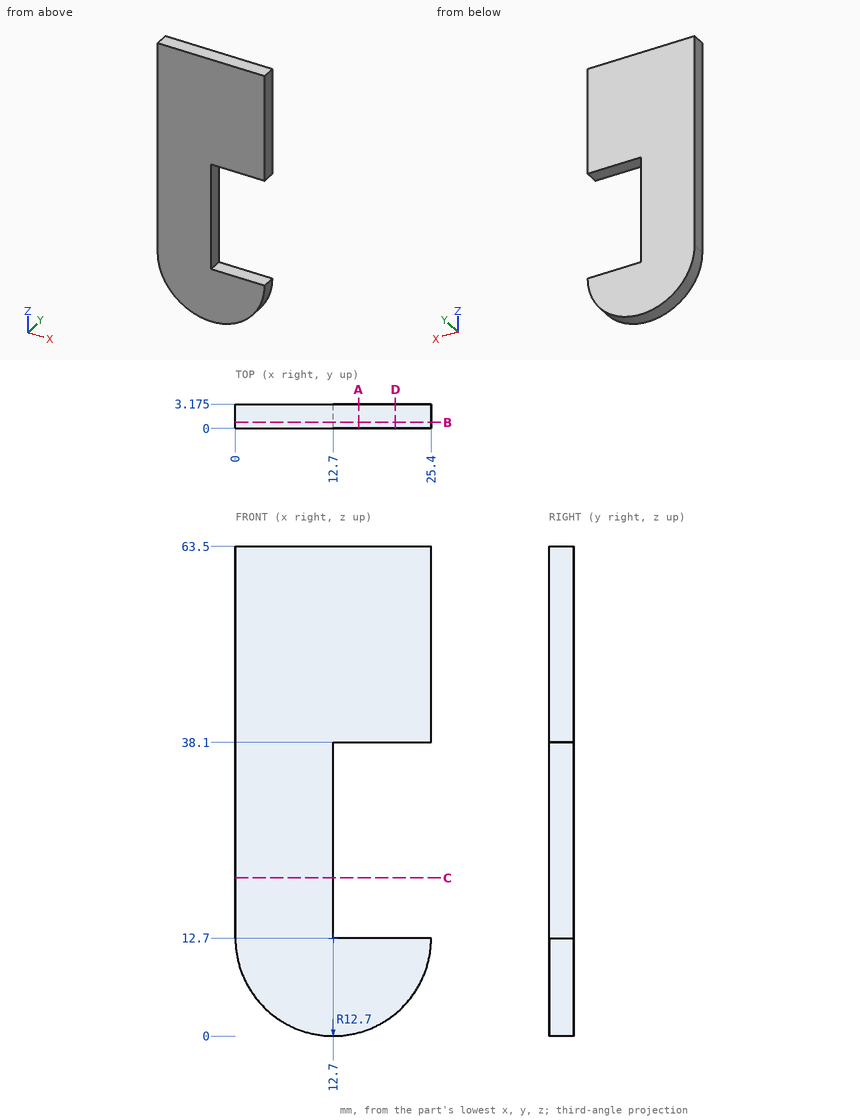
Source: three-view drawing plus pictorial views. Frame: mm from the lowest corner of the part. Round coordinates to 2 decimals unless told otherwise and drop trailing zeros. Order: outer loops, then holes, each group sorted by start corner. A loop starts at its lowest first (then second) coordinate and runs counter-clockwise, first axis right, second up. Notation, with made-up numbers: (83.25, 52) -> (125.25, 52) arc R12 cw to (125.25, 56) -> close; hole circle Ø8 at (64.5, 83). An arc over 180 degrees is marked (long way). Use one line per item in the form item = value.
(1) Ray query, probe 1 along Z at (x, y) = (19, 2.05); probe 2 along Z at (x, y) = (14, 1.4); probe 3 along X at (y, z) = (0.9, 15). Return the intervals inside material, ascending. Write a range as [from, to].
Results list:
probe_1 = [1.67, 12.7], [38.1, 63.5]
probe_2 = [0.07, 12.7], [38.1, 63.5]
probe_3 = [0, 12.7]
(2) Section A-A on x = 16. Return loops of the section in (y, z) (3 decimals), and give its area (3 significant figures).
Results list:
outline = (0, 0.436) -> (3.175, 0.436) -> (3.175, 12.7) -> (0, 12.7) -> close; (0, 38.1) -> (3.175, 38.1) -> (3.175, 63.5) -> (0, 63.5) -> close
area = 120 mm^2
(3) Section C-C on z = 20.5. Return loops of the section in (x, y) (3 decimals), and give its area (3 significant figures).
Results list:
outline = (0, 0) -> (12.7, 0) -> (12.7, 3.175) -> (0, 3.175) -> close
area = 40.3 mm^2
(4) Section B-B on y = 0.8. Return loops of the section in (x, z).
Results list:
outline = (0, 12.7) arc R12.7 ccw to (25.4, 12.7) -> (12.7, 12.7) -> (12.7, 38.1) -> (25.4, 38.1) -> (25.4, 63.5) -> (0, 63.5) -> close
(5) Section D-D on x = 20.75. Return loops of the section in (y, z) (3 decimals).
Results list:
outline = (0, 2.877) -> (3.175, 2.877) -> (3.175, 12.7) -> (0, 12.7) -> close; (0, 38.1) -> (3.175, 38.1) -> (3.175, 63.5) -> (0, 63.5) -> close
(6) First-contact query: pin 1 Ø1 at (y, z) = (2.5, 35.5) entering from +X; pin 2 Ø1.6 at (x, y) = (21, 1) entering from -Z. Flat tips, straight axial feed; report the tip coordinate or a pass-through.
Results list:
pin_1 = 12.7
pin_2 = 2.45
